Part model, mm, in its own coordinate system. Face numbers are marked on the shaded views. Round coordinates to 2 decimals unless told otherwise and drop trailing zeros. Loops run counter-clockwise (first coordinate to the right, second up) from the corner with the lowest first, then second, coordinate; pieces in that order, holes last. Notation, with made-up numbers: M 27,-30.5 L 83,-30.5 A32 ccw 83,5.5 Z; hole C -8.75,54.5 d4. An arc over 180 degrees is marked long. Answer as CSV lines item,"result". Start each with the question number.
Item 1: Band-saw the part on C-C (y = 46). Give the cut face in (x, z), and give its area (3 significant figures).
Item 2: Band-saw the part on A-A (x = 0). Give the cut face in (y, z), and give its area (3 significant figures).
Item 3: Mould opens along X. For the marked faces 1, 2 and 3 say: pulls with the +X half, pulls with the -X half, needs draft (parallel to the pull), parting line crosses it, or undercut.
Item 4: Band-saw the part on D-D (z = -24.5). Give the cut face in (x, y), and give its area (3 significant figures).
Item 5: Wall check: line 1 (X direction, y = 54.75, z = 30); line 2 (X direction, y = 18.5, z = 0); line 3 (Y direction, x = 3.25, z = 31). Give the ranges that are in metal, low to high.
Item 6: Band-saw the part on B-B (z = -38.5). Give the cut face in (x, y), and give its area (3 significant figures).
Item 7: Drop flat-ended pins along their axis: pin 1 Ø6.5 at (x, z) = (0, 30) entering from +Y; pin 2 Ø8 at (x, z) = (0, -40) entering from +Y; pin 3 Ø1.5 at (x, y) = (-1.5, 25) entering from +Z; pin 4 Ø9 at (x, z) = (-3.5, 13) entering from -Y. Give the stop position or say it passes through.
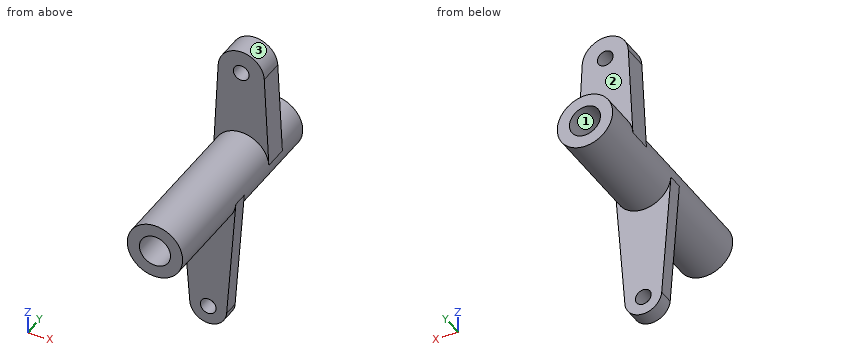
```python
from build123d import *

# Parameters (mm, degrees)
SKETCH_1_R      = 9
SKETCH_1_R_2    = 5.05
EXTRUDE_1_DEPTH = 71
SKETCH_2_R      = 2.55
EXTRUDE_2_DEPTH = 2.5
SKETCH_3_R      = 2.55
EXTRUDE_3_DEPTH = 4


with BuildPart() as part:
    # 草图1 → 凸台-拉伸1 (new body)
    with BuildSketch(Plane(origin=(0, 0, 0), x_dir=(1, 0, 0), z_dir=(0, 1, 0))):
        with Locations(Location((0, 0, 0), (0, 0, 270))):
            Circle(SKETCH_1_R)
        with Locations(Location((0, 0, 0), (0, 0, 270))):
            Circle(SKETCH_1_R_2, mode=Mode.SUBTRACT)
    extrude(amount=EXTRUDE_1_DEPTH)

    # 草图2 → 凸台-拉伸2 (add, symmetric)
    with BuildSketch(Plane(origin=(0, 34, 0), x_dir=(1, 0, 0), z_dir=(0, 1, 0))):
        with BuildLine():
            ThreePointArc((-8.974651804, 0.675), (0, 9), (8.974651804, 0.675))
            Line((8.974651804, 0.675), (5.983101203, 40.45))
            ThreePointArc((5.983101203, 40.45), (0, 46), (-5.983101203, 40.45))
            Line((-5.983101203, 40.45), (-8.974651804, 0.675))
        make_face()
        with Locations(Location((0, 40, 0), (0, 0, 270))):
            Circle(SKETCH_2_R, mode=Mode.SUBTRACT)
    extrude(amount=EXTRUDE_2_DEPTH, both=True)

    # 草图3 → 凸台-拉伸3 (add, symmetric)
    with BuildSketch(Plane(origin=(0, 55, 0), x_dir=(1, 0, 0), z_dir=(0, 1, 0))):
        with BuildLine():
            ThreePointArc((8.98874296, -0.45), (0, -9), (-8.98874296, -0.45))
            Line((-8.98874296, -0.45), (-7.490619133, -30.375))
            ThreePointArc((-7.490619133, -30.375), (0, -37.5), (7.490619133, -30.375))
            Line((7.490619133, -30.375), (8.98874296, -0.45))
        make_face()
        with Locations(Location((0, -30, 0), (0, 0, 270))):
            Circle(SKETCH_3_R, mode=Mode.SUBTRACT)
    extrude(amount=EXTRUDE_3_DEPTH, both=True)


solid = part.part
```
Answer block:
1,outline,"C 0,0 d18; hole C 0,0 d10.1"
1,area,"174 mm^2"
2,outline,"M 0,-9 L 31.5,-9 L 31.5,-37.45 L 36.5,-37.45 L 36.5,-9 L 71,-9 L 71,-5.05 L 0,-5.05 Z; M 0,5.05 L 71,5.05 L 71,9 L 59,9 L 59,27.45 L 51,27.45 L 51,9 L 0,9 Z; M 31.5,-46 L 36.5,-46 L 36.5,-42.55 L 31.5,-42.55 Z; M 51,32.55 L 59,32.55 L 59,37.5 L 51,37.5 Z"
2,area,"908 mm^2"
3,face 1,"undercut"
3,face 2,"needs draft"
3,face 3,"parting line crosses it"
4,outline,"M -7.18,31.5 L 7.18,31.5 L 7.18,36.5 L -7.18,36.5 Z"
4,area,"71.8 mm^2"
5,line 1,"x = -7.51 to -2.55, 2.55 to 7.51"
5,line 2,"x = -9 to -5.05, 5.05 to 9"
5,line 3,"y = 51 to 59"
6,outline,"M -6.13,31.5 L -2.06,31.5 L -2.06,36.5 L -6.13,36.5 Z; M 2.06,31.5 L 6.13,31.5 L 6.13,36.5 L 2.06,36.5 Z"
6,area,"40.7 mm^2"
7,pin 1,"stops at y = 59"
7,pin 2,"stops at y = 36.5"
7,pin 3,"stops at z = 8.97"
7,pin 4,"stops at y = 0"
